The model under review builds one solid part; all positions refer to its coordinate system, in mm. Face numbers are marked on the shaded views. A direction names the side the tool comes from. Round coordinates to 2 decimals unless told otherwise and drop trailing zeros. Order: outer loops, then holes, each group sorted by start corner. A loop starts at its lowest first (then second) coordinate and runs counter-clockwise, first axis right, second up. Notation, with made-up numbers: M 20.25,-10.5 L 45.25,-10.5 A25 cw 45.25,26.5 Z; hole C 76,76.5 d3. An arc over 180 degrees is marked long. Answer as a JSON object with one key per item and string values. Group by question number.
1. To check wall thickness, follow probe 1 along Y at (x, z) = (0, 0.8) (3 decimals); probe 2 along Y at (x, z) = (0, 1.2); probe 3 along X at (y, z) = (0, 0.75) (3 decimals). State the ranges of each line that lie inside material, in increasing order. Write a range as [from, to].
2. Mouldability with a two-part tool opening along Y and no side actions: class the marked faces 4, 5 and 6 as released by +Y, released by -Y, zero draft, split by the parting line, or undercut.
3. Add section A-A on z = 8.5. State the section outline as (x, y) points, and give its area (3 significant figures).
4. Clearance check with flat-ended pins moving along their axes: P1, Ø0.8, axis at x = -5.5, y = 0, coming from the +Z side; P2, Ø3, axis at x = -5, z = 8, coming from the -Y side; P3, Ø1.5, axis at x = 5, z = 2.5, coming from the -Y side; P4, Ø4.5, axis at x = 0, y = 0, coming from the -Z side. State where each tip first meets the part, or that it passes through.
5. Machinability: for the marked faces 1, 2 and 3, which of the approach directions +Z, -Z, +X, -X, +Y, -Y give a long, thin tool a straight path to every point of the face, cutting with its end or side? Answer none if there is none.
6. Add section B-B on z = 6.5. Give the number of separate pieces and of enclosed holes in the cut face, and give its area (3 significant figures).
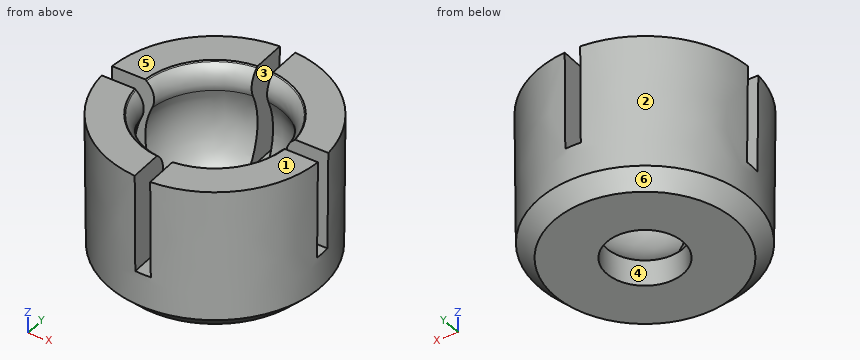
```python
from build123d import *

# Parameters (mm, degrees)
POCKET_DEPTH = 6.413333


with BuildPart() as part:
    # Sketch001 → Revolution (revolve)
    with BuildSketch(Plane.XZ):
        with BuildLine():
            ThreePointArc((-4.423636, 7.90675), (-4.652325, 4.430289), (-2.5, 1.690658))
            Line((-2.5, 0), (-2.5, 1.690658))
            Line((-5.925, 0), (-2.5, 0))
            Line((-6.925, 1), (-5.925, 0))
            Line((-6.925, 1), (-7, 9.62))
            Line((-7, 9.62), (-4.87, 9.62))
            Line((-4.87, 9.62), (-4.793396, 9.555721))
            ThreePointArc((-4.423636, 7.90675), (-4.329753, 8.793744), (-4.793396, 9.555721))
        make_face()
    revolve(axis=Axis((0, 0, 0), (0, 0, 1)))

    # Sketch (on Face6 of Revolution) → Pocket (cut)
    with BuildSketch(Plane(origin=(0, 0, 9.62), x_dir=(-1, 0, 0), z_dir=(0, 0, 1))):
        Polygon((-0.5, 14.35), (-0.5, 0.5), (-14.35, 0.5), (-14.35, -0.5), (-0.5, -0.5), (-0.5, -14.35), (0.5, -14.35), (0.5, -0.5), (14.35, -0.5), (14.35, 0.5), (0.5, 0.5), (0.5, 14.35), align=None)
    extrude(amount=-POCKET_DEPTH, mode=Mode.SUBTRACT)


solid = part.part
```
Recorded:
{
 "1": {"probe 1": "y = [-6.725, -2.5], [2.5, 6.725]", "probe 2": "y = [-6.93, -2.5], [2.5, 6.93]", "probe 3": "x = [-6.675, -2.5], [2.5, 6.675]"},
 "2": {"face 4": "undercut", "face 5": "zero draft", "face 6": "split by the parting line"},
 "3": {"outline": "M -6.97,-0.5 A6.99 ccw -0.5,-6.97 L -0.5,-4.27 A4.3 cw -4.27,-0.5 Z; M -6.97,0.5 L -4.27,0.5 A4.3 cw -0.5,4.27 L -0.5,6.97 A6.99 ccw Z; M 0.5,-6.97 A6.99 ccw 6.97,-0.5 L 4.27,-0.5 A4.3 cw 0.5,-4.27 Z; M 0.5,4.27 A4.3 cw 4.27,0.5 L 6.97,0.5 A6.99 ccw 0.5,6.97 Z", "area": "84.7 mm²"},
 "4": {"P1": "stops at z = 3.21", "P2": "stops at y = -6.05", "P3": "stops at y = -5.48", "P4": "passes through"},
 "5": {"face 1": "+Z, +X, -X, +Y, -Y", "face 2": "-Z", "face 3": "+Z, +Y, -Y"},
 "6": {"separate pieces": "4", "enclosed holes": "0", "area": "70.9 mm²"}
}
